from build123d import *

# Parameters (mm, degrees)
SKETCH_R        = 5
SKETCH_R_2      = 3.2
PAD_DEPTH       = 15
SKETCH002_R     = 6.1
POCKET001_DEPTH = 4
SKETCH003_R     = 11.1
POCKET_DEPTH    = 7.4
FILLET_R        = 4
CHAMFER_SIZE    = 0.4
CHAMFER001_SIZE = 0.4


with BuildPart() as part:
    # Sketch → Pad (new body)
    with BuildSketch(Plane.XY):
        Polygon((20, 30), (20, 51), (62.3, 51), (62.3, 30), (82.3, 30), (82.3, 0), (0, 0), (0, 30), align=None)
        with Locations((41.15, 29.85)):
            Circle(SKETCH_R, mode=Mode.SUBTRACT)
        with Locations((11.15, 10)):
            Circle(SKETCH_R_2, mode=Mode.SUBTRACT)
        with Locations((31.15, 10)):
            Circle(SKETCH_R_2, mode=Mode.SUBTRACT)
        with Locations((51.15, 10)):
            Circle(SKETCH_R_2, mode=Mode.SUBTRACT)
        with Locations((71.15, 10)):
            Circle(SKETCH_R_2, mode=Mode.SUBTRACT)
    extrude(amount=PAD_DEPTH)

    # Sketch002 → Pocket001 (cut)
    with BuildSketch(Plane(origin=(0, 0, 0), x_dir=(1, 0, 0), z_dir=(0, 0, -1))):
        with Locations((11.15, -10)):
            Circle(SKETCH002_R)
        with Locations((31.15, -10)):
            Circle(SKETCH002_R)
        with Locations((51.15, -10)):
            Circle(SKETCH002_R)
        with Locations((71.15, -10)):
            Circle(SKETCH002_R)
    extrude(amount=-POCKET001_DEPTH, mode=Mode.SUBTRACT)

    # Sketch003 (on Face5 of Pocket001) → Pocket (cut)
    with BuildSketch(Plane.XY.offset(15)):
        with Locations((41.15, 29.85)):
            Circle(SKETCH003_R)
    extrude(amount=-POCKET_DEPTH, mode=Mode.SUBTRACT)

    # Fillet
    fillet_edges = [part.edges().sort_by_distance(p)[0] for p in [
        (82.3, 0, 7.5),
        (0, 0, 7.5),
        (0, 30, 7.5),
        (20, 30, 7.5),
        (20, 51, 7.5),
        (62.3, 51, 7.5),
        (62.3, 30, 7.5),
        (82.3, 30, 7.5),
    ]]
    fillet(fillet_edges, radius=FILLET_R)

    # Chamfer
    chamfer_edges = [part.edges().sort_by_distance(p)[0] for p in [
        (20, 40.5, 0),
        (18.828427, 31.171573, 0),
        (21.171573, 49.828427, 0),
        (10, 30, 0),
        (41.15, 51, 0),
        (1.171573, 28.828427, 0),
        (61.128427, 49.828427, 0),
        (0, 15, 0),
        (62.3, 40.5, 0),
        (1.171573, 1.171573, 0),
        (63.471573, 31.171573, 0),
        (41.15, 0, 0),
        (72.3, 30, 0),
        (81.128427, 1.171573, 0),
        (81.128427, 28.828427, 0),
        (82.3, 15, 0),
        (65.05, 10, 0),
        (45.05, 10, 0),
        (25.05, 10, 0),
        (5.05, 10, 0),
        (36.15, 29.85, 0),
    ]]
    chamfer(chamfer_edges, length=CHAMFER_SIZE)

    # Chamfer001
    chamfer001_edges = [part.edges().sort_by_distance(p)[0] for p in [
        (20, 40.5, 15),
        (18.828427, 31.171573, 15),
        (21.171573, 49.828427, 15),
        (10, 30, 15),
        (41.15, 51, 15),
        (1.171573, 28.828427, 15),
        (61.128427, 49.828427, 15),
        (0, 15, 15),
        (62.3, 40.5, 15),
        (1.171573, 1.171573, 15),
        (63.471573, 31.171573, 15),
        (41.15, 0, 15),
        (72.3, 30, 15),
        (81.128427, 1.171573, 15),
        (81.128427, 28.828427, 15),
        (82.3, 15, 15),
        (67.95, 10, 15),
        (47.95, 10, 15),
        (27.95, 10, 15),
        (7.95, 10, 15),
        (30.05, 29.85, 15),
    ]]
    chamfer(chamfer001_edges, length=CHAMFER001_SIZE)


solid = part.part
Could you check a few things on this model? Use its own coordinates, in mm. A direction names the side the tool comes from. Give positions to 0.01 mm unless a question says otherwise; leave off trailing zeros. Order: outer loops, then holes, each group sorted by start corner. A loop starts at its lowest first (then second) coordinate and runs counter-clockwise, first axis right, second up.
1. I need wall thicknesses on L1, parallel to X at y = 10, z = 7.5; L2, parallel to X at y = 10, z = 1.9; L3, parallel to Y at x = 31.15, z = 10.25. Which ranges of each line are inside material? Lowest first, please.
2. We'd pull the mould along Y, two halves only. Please class faces 4 (the conical face through (1.407, 1.349, 0.108)), 5 (the cylindrical face through (63.441, 31.203, 7.599)), 6 (the cylindrical face through (36.8, 12.3, 2.2)): pulls with the +Y half, pulls with the -Y half, needs draft (parallel to the pull), parting line crosses it, or undercut.
3. Will these pins go through, and if not, where does the flat tip stop? P1, Ø1, axis at x = 16.5, z = 3.5, coming from the +Y side; P2, Ø8, axis at x = 64.5, z = 4.5, coming from the +Y side; P3, Ø13, axis at x = 41.15, y = 29.85, coming from the +Z side; P4, Ø4, axis at x = 51.15, y = 10, coming from the +Z side.
4. Suppose I cut it at A-A (x = 11.15). List the corners of the cut face in (y, z) for me, plus the area to 3 significant figures.
5. Suppose I cut it at B-B (z = 11.5). List the corners of the cut face in (x, y) for me.
6. Suppose I cut it at C-C (y = 44). List the corners of the cut face in (x, z) for me, plus the area to 3 significant figures.
7. For faces 1 (the cylindrical face through (47.12, 39.21, 11.15)), 2 (the flat face through (14, 13, 4)), 3 (the conical face through (80.893, 28.651, 14.892)), which set-ups out of +Z, -Z, +X, -X, +Y, -Y let a thin tool reach every point of the face, with its end or its side?
Solved:
1. L1: x = 0 to 7.95, 14.35 to 27.95, 34.35 to 47.95, 54.35 to 67.95, 74.35 to 82.3
1. L2: x = 0 to 5.05, 17.25 to 25.05, 37.25 to 45.05, 57.25 to 65.05, 77.25 to 82.3
1. L3: y = 0 to 6.8, 13.2 to 25.03, 34.67 to 51
2. face 4: pulls with the -Y half
2. face 5: pulls with the +Y half
2. face 6: undercut
3. P1: stops at y = 30.13
3. P2: stops at y = 50.34
3. P3: stops at z = 7.6
3. P4: passes through
4. outline: (0, 0.4) - (0.4, 0) - (3.5, 0) - (3.9, 0.4) - (3.9, 4) - (6.8, 4) - (6.8, 14.6) - (6.4, 15) - (0.4, 15) - (0, 14.6) - close; (13.2, 4) - (16.1, 4) - (16.1, 0.4) - (16.5, 0) - (29.6, 0) - (30, 0.4) - (30, 14.6) - (29.6, 15) - (13.6, 15) - (13.2, 14.6) - close
4. area: 330 mm2
5. outline: (0, 4) arc R4 ccw to (4, 0) - (78.3, 0) arc R4 ccw to (82.3, 4) - (82.3, 26) arc R4 ccw to (78.3, 30) - (66.3, 30) arc R4 cw to (62.3, 34) - (62.3, 47) arc R4 ccw to (58.3, 51) - (24, 51) arc R4 ccw to (20, 47) - (20, 34) arc R4 cw to (16, 30) - (4, 30) arc R4 ccw to (0, 26) - close; hole circle Ø6.4 at (11.15, 10); hole circle Ø6.4 at (31.15, 10); hole circle Ø22.2 at (41.15, 29.85); hole circle Ø6.4 at (51.15, 10); hole circle Ø6.4 at (71.15, 10)
6. outline: (20, 0.4) - (20.4, 0) - (61.9, 0) - (62.3, 0.4) - (62.3, 14.6) - (61.9, 15) - (20.4, 15) - (20, 14.6) - close
6. area: 634 mm2
7. face 1: +Z
7. face 2: -Z
7. face 3: +Z, +X, +Y
